```python
from build123d import *

# Parameters (mm, degrees)
CROQUIS1_W              = 15
CROQUIS1_H              = 15
SALIENTE_EXTRUIR1_DEPTH = 65
CORTAR_EXTRUIR1_DEPTH   = 68.12860791


with BuildPart() as part:
    # Croquis1 → Saliente-Extruir1 (new, symmetric)
    with BuildSketch(Plane(origin=(0, 0, 0), x_dir=(0, 0, -1), z_dir=(1, 0, 0))):
        Rectangle(CROQUIS1_W, CROQUIS1_H)
    extrude(amount=SALIENTE_EXTRUIR1_DEPTH, both=True)

    # Croquis2 → Cortar-Extruir1 (cut, through all)
    with BuildSketch(Plane.XZ.offset(7.5)):
        with BuildLine():
            Line((44.847129428, 2.531795375), (55.614029525, 2.531795375))
            ThreePointArc((55.614029525, 2.531795375), (58.1458249, 0), (55.614029525, -2.531795375))
            Line((55.614029525, -2.531795375), (44.847129428, -2.531795375))
            ThreePointArc((44.847129428, -2.531795375), (42.315334053, 0), (44.847129428, 2.531795375))
        make_face()
    extrude(amount=-CORTAR_EXTRUIR1_DEPTH, mode=Mode.SUBTRACT)


solid = part.part
```
Input: part model. Units: mm. Frame: model coordinates. A direction names the side the tool comes from. Round coordinates to 2 decimals unless told otherwise and drop trailing zeros. Loops run counter-clockwise (first coordinate to the right, second up) from the corner with the lowest first, then second, coordinate; pieces in that order, holes last. Notation, with made-up numbers: (-6, 43) -> (31, 43) arc R18 cw to (31, 69) -> close; hole circle Ø11 at (86, 3). An arc over 180 degrees is marked (long way). Write each question's results on one line, items separated by ' | '.
1. Section B-B (y = 1.75). Return loops of the section in (x, z).
Geometry results:
outline: (-65, -7.5) -> (65, -7.5) -> (65, 7.5) -> (-65, 7.5) -> close; hole (44.85, -2.53) -> (55.61, -2.53) arc R2.53 ccw to (55.61, 2.53) -> (44.85, 2.53) arc R2.53 ccw to start
2. Section A-A (z = 0). Return loops of the section in (x, y).
Geometry results:
outline: (-65, -7.5) -> (42.32, -7.5) -> (42.32, 7.5) -> (-65, 7.5) -> close; (58.15, -7.5) -> (65, -7.5) -> (65, 7.5) -> (58.15, 7.5) -> close
3. Set-up query: faces 1 (the face through (50, 0, -2.532)), 2 (the face through (1, 7.5, 0)). Return all of +Z, -Z, +X, -X, +Y, -Y with unobstructed straight access to the full face (end or side cutting, diameter ignored); none if empty.
Geometry results:
face 1: +Y, -Y | face 2: +Z, -Z, +X, -X, +Y
4. Ray query, line 1 (Z direction, x = 53.5, y = 4); line 2 (X direction, y = -5, z = 2); line 3 (X direction, y = 3.75, z = -2.25). Return the intervals inside material, ascending. Write a range as from..to.
Geometry results:
line 1: -7.5..-2.53, 2.53..7.5 | line 2: -65..43.29, 57.17..65 | line 3: -65..43.69, 56.77..65
5. Mould query, pull axis X, two halves, no side actions, for faces 3 (the face through (50, 0, 2.532)), 4 (the face through (-65, 0, 0)), 5 (the face through (1, 0, 7.5)), 6 (the face through (42.316, -0.105, -0.056)). Classes: +X half, -X half, draft (parallel to the pull), parting line (faces both ways), or undercut.
Geometry results:
face 3: undercut | face 4: -X half | face 5: draft | face 6: undercut
6. Section C-C (x = 50). Return loops of the section in (y, z).
Geometry results:
outline: (-7.5, -7.5) -> (7.5, -7.5) -> (7.5, -2.53) -> (-7.5, -2.53) -> close; (-7.5, 2.53) -> (7.5, 2.53) -> (7.5, 7.5) -> (-7.5, 7.5) -> close
